Geometry: final body of the model. Coordinates: model frame, mm. Coordinates: 2 decimals unless noted, no trailing zeros. Loops run counter-clockwise (first coordinate to the right, second up) from the corner with the lowest first, then second, coordinate; pieces in that order, holes last. Notation, with made-up numbers: (-12, -9.75) - (40, -9.75) arc R26 cw to (40, 14.25) - close; hole circle Ø9 at (43.25, -39). An arc over 180 degrees is marked (long way). Answer in a Markdown table with one row per item.
from build123d import *

# Parameters (mm, degrees)
SKETCH_1_W          = 55
SKETCH_1_H          = 30
EXTRUDE_1_DEPTH     = 2
SKETCH_2_R          = 1.525
CUT_EXTRUDE_1_DEPTH = 2
FILLET_1_R          = 3
CUT_EXTRUDE_2_DEPTH = 2
FILLET_2_R          = 1


with BuildPart() as part:
    # 草图1 → 凸台-拉伸1 (new body)
    with BuildSketch(Plane(origin=(0, 0, 0), x_dir=(1, 0, 0), z_dir=(0, 1, 0))):
        Rectangle(SKETCH_1_W, SKETCH_1_H)
    extrude(amount=EXTRUDE_1_DEPTH)

    # 草图2 → 切除-拉伸1 (cut)
    with BuildSketch(Plane(origin=(0, 2, 0), x_dir=(1, 0, 0), z_dir=(0, 1, 0))):
        with Locations((-23.5, 10)):
            Circle(SKETCH_2_R)
        with Locations((-23.5, -10)):
            Circle(SKETCH_2_R)
        with Locations((23.5, -10)):
            Circle(SKETCH_2_R)
        with Locations((23.5, 10)):
            Circle(SKETCH_2_R)
    extrude(amount=-CUT_EXTRUDE_1_DEPTH, mode=Mode.SUBTRACT)

    # 圆角1
    fillet_1_edges = [part.edges().sort_by_distance(p)[0] for p in [
        (27.5, 1, 15),
        (-27.5, 1, 15),
        (-27.5, 1, -15),
        (27.5, 1, -15),
    ]]
    fillet(fillet_1_edges, radius=FILLET_1_R)

    # 草图3 → 切除-拉伸2 (cut)
    with BuildSketch(Plane(origin=(0, 2, 0), x_dir=(1, 0, 0), z_dir=(0, 1, 0))):
        Polygon((-15.75, 10), (15.75, 10), (0, 1), align=None)
        Polygon((-15.75, 6.544746679), (-15.75, -6.544746679), (-4.296693311, 0), align=None)
        Polygon((-15.75, -10), (15.75, -10), (0, -1), align=None)
        Polygon((15.75, 6.544746679), (15.75, -6.544746679), (4.296693311, 0), align=None)
    extrude(amount=-CUT_EXTRUDE_2_DEPTH, mode=Mode.SUBTRACT)

    # 圆角2
    fillet_2_edges = [part.edges().sort_by_distance(p)[0] for p in [
        (15.75, 1, 10),
        (0, 1, 1),
        (-15.75, 1, 10),
        (-15.75, 1, 6.544746679),
        (-4.296693311, 1, 0),
        (-15.75, 1, -6.544746679),
        (15.75, 1, 6.544746679),
        (15.75, 1, -6.544746679),
        (4.296693311, 1, 0),
        (15.75, 1, -10),
        (-15.75, 1, -10),
        (0, 1, -1),
    ]]
    fillet(fillet_2_edges, radius=FILLET_2_R)


solid = part.part
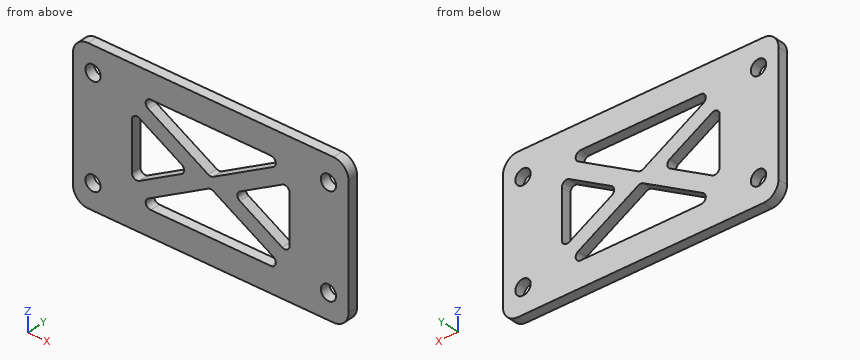
(1) Cut plane D-D on x = 6.5. Output: boundary loops of the cut face in (y, z), then the cut area to 3 significant figures.
Verdict:
| item | result |
|---|---|
| outline | (0, -15) - (2, -15) - (2, -10) - (0, -10) - close; (0, -4.71) - (2, -4.71) - (2, -1.26) - (0, -1.26) - close; (0, 1.26) - (2, 1.26) - (2, 4.71) - (0, 4.71) - close; (0, 10) - (2, 10) - (2, 15) - (0, 15) - close |
| area | 33.8 mm² |
(2) Cut plane B-B on z = 4. Output: boundary loops of the cut face in (x, y), then the cut area to 3 significant figures.
Verdict:
| item | result |
|---|---|
| outline | (-27.5, 0) - (-15.75, 0) - (-15.75, 2) - (-27.5, 2) - close; (-11.3, 0) - (-5.25, 0) - (-5.25, 2) - (-11.3, 2) - close; (5.25, 0) - (11.3, 0) - (11.3, 2) - (5.25, 2) - close; (15.75, 0) - (27.5, 0) - (27.5, 2) - (15.75, 2) - close |
| area | 71.2 mm² |
(3) Ray query, probe 1 along Z at (x, y) = (23.5, 1.9) (3 decimals); probe 2 along Z at (x, y) = (-7.5, 0.6); probe 3 along X at (y, z) = (1.9, -9.5). Return the intervals inside material, ascending.
Verdict:
| item | result |
|---|---|
| probe 1 | z = -15 to -11.525, -8.475 to 8.475, 11.525 to 15 |
| probe 2 | z = -15 to -10, -5.29 to -1.83, 1.83 to 5.29, 10 to 15 |
| probe 3 | x = -27.5 to -24.94, -22.06 to -12.85, 12.85 to 22.06, 24.94 to 27.5 |
(4) Cut plane A-A on x = -23.5. Output: boundary loops of the cut face in (y, z) (3 decimals).
Verdict:
| item | result |
|---|---|
| outline | (0, -15) - (2, -15) - (2, -11.525) - (0, -11.525) - close; (0, -8.475) - (2, -8.475) - (2, 8.475) - (0, 8.475) - close; (0, 11.525) - (2, 11.525) - (2, 15) - (0, 15) - close |
(5) Cut plane C-C on y = 0.6. State how many separate pieces and enclosed holes the cut face has, then the cut area to 3 significant figures.
Verdict:
| item | result |
|---|---|
| separate pieces | 1 |
| enclosed holes | 8 |
| area | 1,190 mm² |
(6) First-contact query: pin 1 Ø2.5 at (x, z) = (23.5, 10) entering from +Y. Flat tip, straight axial feed; report the tip coordinate or a pass-through.
Verdict:
| item | result |
|---|---|
| pin 1 | passes through |
